```python
from build123d import *

# Parameters (mm, degrees)
F0_W     = 127.008882
F0_H     = 76.652937
F1_DEPTH = 38.1
F2_T     = -2.54
F3_W     = 118.68491
F3_H     = 67.936881
F4_DEPTH = 4.7752


with BuildPart() as f1:
    # F0 (on Front) → F1 (new body)
    with BuildSketch(Plane.XZ):
        with Locations((3.217185, 6.294493)):
            Rectangle(F0_W, F0_H)
    extrude(amount=F1_DEPTH)

    # F2
    f2_openings = [f1.faces().sort_by_distance(p)[0] for p in [
        (3.217185, 0, 6.294493),
    ]]
    offset(amount=F2_T, openings=f2_openings)

    # F3 (on face) → F4 (join)
    with BuildSketch(Plane.XZ.offset(38.1)):
        with Locations((3.130339, 6.138873)):
            Rectangle(F3_W, F3_H)
    extrude(amount=F4_DEPTH)


solid = f1.part
```
Geometry: final body of the model. Coordinates: model frame, mm. A direction names the side the tool comes from. Give positions to 0.01 mm unless a question says otherwise; leave off trailing zeros. Write each loop counter-clockwise with the first axis right and the second up, starting at its lowest first coordinate (ties: lowest second). Pieces come first, ordered by that corner, then holes.
1. Section query C-C, the plane x = 16.5. Return loops of the section in (y, z), then the cut area to 3 significant figures.
2. Section query A-A, the plane z = -19.5. Return loops of the section in (x, y), then the cut area to 3 significant figures.
3. Line query: probe 1 along Z at (x, y) = (-54.5, -23); probe 2 along X at (y, z) = (-27, -4.5); probe 3 along Y at (x, z) = (26, 0). Output: solid intervals per line, ascending.
4. Draft query along X for faces 6 (the flat face through (-57.747, -18, 6)), 7 (the flat face through (62.473, -40, 6)), 8 (the flat face through (-16, 0, 43)). Return one class per face: released by +X, released by -X, zero draft, split by the parting line, or undercut.
5. Reachability of faces 1 (the flat face through (2, -40, 40.107)), 2 (the flat face through (2, -35.56, 7)), 3 (the flat face through (2, -42.875, 7)), 4 (the flat face through (2, -40, -27.83)), 5 (the flat face through (-56.212, -40, 6)) from +Z, -Z, +X, -X, +Y, -Y: full face, straight path, thin tool, end or side. Return the list, or none.
6. Pin query (flat end, axial travel): P1, Ø4, axis at x = -26, y = -40.5, coming from the +Z side; P2, Ø5.5, axis at y = -41, z = -8.5, coming from the +X side; P3, Ø12, axis at x = 6, z = 21.5, coming from the +Y side; P4, Ø5.5, axis at x = 26, y = -39.5, coming from the -Z side. Return the tip coordinate at first contact, or that it passes through.
7. Section query B-B, the plane y = -5. Return loops of the section in (x, z).
Computed:
1. outline: (-42.88, -27.83) - (-38.1, -27.83) - (-38.1, -32.03) - (0, -32.03) - (0, -29.49) - (-35.56, -29.49) - (-35.56, 42.08) - (0, 42.08) - (0, 44.62) - (-38.1, 44.62) - (-38.1, 40.11) - (-42.88, 40.11) - close
1. area: 700 mm2
2. outline: (-60.29, -38.1) - (-56.21, -38.1) - (-56.21, -42.88) - (62.47, -42.88) - (62.47, -38.1) - (66.72, -38.1) - (66.72, 0) - (64.18, 0) - (64.18, -35.56) - (-57.75, -35.56) - (-57.75, 0) - (-60.29, 0) - close
2. area: 1,070 mm2
3. probe 1: z = -32.03 to -29.49, 42.08 to 44.62
3. probe 2: x = -60.29 to -57.75, 64.18 to 66.72
3. probe 3: y = -42.88 to -35.56
4. face 6: undercut
4. face 7: released by +X
4. face 8: zero draft
5. face 1: +Z, +X, -X, -Y
5. face 2: +Y
5. face 3: +Z, -Z, +X, -X, -Y
5. face 4: -Z, +X, -X, -Y
5. face 5: +Z, -Z, -X, -Y
6. P1: stops at z = 40.11
6. P2: stops at x = 62.47
6. P3: stops at y = -35.56
6. P4: stops at z = -32.03
7. outline: (-60.29, -32.03) - (66.72, -32.03) - (66.72, 44.62) - (-60.29, 44.62) - close; hole (-57.75, -29.49) - (64.18, -29.49) - (64.18, 42.08) - (-57.75, 42.08) - close
